The model under review builds one solid part; all positions refer to its coordinate system, in mm. A direction names the side the tool comes from. Round coordinates to 2 decimals unless told otherwise and drop trailing zeros. Write each loop counter-clockwise with the first axis right and the second up, starting at its lowest first coordinate (ties: lowest second). Pieces come first, ordered by that corner, then holes. Notation, with made-up numbers: (73, 24) - (78, 24) arc R16 ccw to (78, 53) - close; hole circle Ø4 at (0, 65). An arc over 180 degrees is marked (long way). One line per question, with ' | ' between items. Start each with the question number.
```python
from build123d import *

# Parameters (mm, degrees)
F0_W     = 42
F0_H     = 42
F1_DEPTH = 500


with BuildPart() as f1:
    # F0 (on Right) → F1 (new body, symmetric)
    with BuildSketch(Plane.YZ):
        with BuildLine():
            Line((21, 25), (-21, 25))
            ThreePointArc((-21, 25), (-23.828427, 23.828427), (-25, 21))
            Line((-25, 21), (-25, -21))
            ThreePointArc((-25, -21), (-23.828427, -23.828427), (-21, -25))
            Line((-21, -25), (21, -25))
            ThreePointArc((21, -25), (23.828427, -23.828427), (25, -21))
            Line((25, -21), (25, 21))
            ThreePointArc((25, 21), (23.828427, 23.828427), (21, 25))
        make_face()
        Rectangle(F0_W, F0_H, mode=Mode.SUBTRACT)
    extrude(amount=F1_DEPTH, both=True)


solid = f1.part
```
1. Machinability: for faces 1 (the face through (7, 0, 21)), 2 (the face through (-500, -23, 0)), which of the approach directions +Z, -Z, +X, -X, +Y, -Y give a long, thin tool a straight path to every point of the face, cutting with its end or side? Answer none if there is none.
2. Add section C-C, the plane x = 434. Write out the cut boundary in (y, z).
3. The part is to be moulded in two halves that separate along Y. For faces 3 (the face through (7, -25, 0)), 4 (the face through (7, 25, 0)), 5 (the face through (500, -23, 0)), 6 (the face through (7, 21, 0)), say which applies: pulls with the +Y half, pulls with the -Y half, needs draft (parallel to the pull), parting line crosses it, or undercut.
4. Wall thickness on line 1 along Y through (x, z) = (289, 12); line 2 along Z through (x, y) = (-174, 22): over which ranges is each line inside the solid? List them lowest first. Write a range as [from, to].
5. Add section A-A, the plane z = -2.5. Write out the cut boundary in (x, y), then the cut area to 3 significant figures.
Geometry check:
1) face 1: +X, -X | face 2: +Z, -Z, -X, +Y, -Y
2) outline: (-25, -21) arc R4 ccw to (-21, -25) - (21, -25) arc R4 ccw to (25, -21) - (25, 21) arc R4 ccw to (21, 25) - (-21, 25) arc R4 ccw to (-25, 21) - close; hole (-21, -21) - (21, -21) - (21, 21) - (-21, 21) - close
3) face 3: pulls with the -Y half | face 4: pulls with the +Y half | face 5: needs draft | face 6: undercut
4) line 1: y = [-25, -21], [21, 25] | line 2: z = [-24.87, 24.87]
5) outline: (-500, -25) - (500, -25) - (500, -21) - (-500, -21) - close; (-500, 21) - (500, 21) - (500, 25) - (-500, 25) - close | area: 8,000 mm2
